CAD build for the part. Positions are in the model's coordinates, mm. Face numbers are marked on the shaded views. A direction names the side the tool comes from. Give positions to 0.01 mm unless a question says otherwise; leave off trailing zeros. Order: outer loops, then holes, each group sorted by start corner. A loop starts at its lowest first (then second) coordinate and runs counter-clockwise, first axis right, second up.
Item 1: Band-saw the part on A-A on x = -6. Give the cut face in (y, z), plus the area to 3 significant figures.
Item 2: Band-saw the part on D-D on x = 15.25. Give the cut face in (y, z).
Item 3: Which spindle directions (+Z, -Z, +X, -X, +Y, -Y) get a long thin tool onto all of the face, cutting with end or side? Do the marked faces 1, 2 and 3. Say none if no direction does.
Item 4: Flat gauge pins, fed straight in: P1, Ø3.5, axis at x = 15, z = 11.5, coming from the -Y side; P2, Ø2, axis at y = -12.5, z = 17.5, coming from the +X side; P3, Ø1.5, axis at x = 15.5, z = 18, coming from the +Y side. Where does each tip first touch, or does it go through?
Item 5: Wall check: L1, parallel to X at y = -0.25, z = 15.5; L2, parallel to X at y = -14.5, z = 23; L3, parallel to X at y = 0.25, z = 6.75. Give the ranges that are in metal, low to high.
Item 6: Band-saw the part on C-C on y = -11.5. Give the cut face in (x, z), plus the area to 3 significant figures.
Item 7: Band-saw the part on B-B on z = 8. Give the cut face in (x, y), plus the area to 3 significant figures.
```python
from build123d import *

# Parameters (mm, degrees)
F1_DEPTH = 25


with BuildPart() as f1:
    # F0 (on Top) → F1 (new body)
    with BuildSketch(Plane.XY):
        with BuildLine():
            ThreePointArc((0, -10.5), (-7.4246212025, 7.4246212025), (10.5, 0))
            Line((10.5, 0), (12, 0))
            ThreePointArc((12, 0), (-8.4852813742, 8.4852813742), (0, -12))
            Line((0, -12), (0, -10.5))
        make_face()
        with BuildLine():
            Line((12, 0), (10.5, 0))
            ThreePointArc((10.5, 0), (10.473041604, -0.7519305564), (10.3923048454, -1.5))
            Line((10.3923048454, -1.5), (11.9058808998, -1.5))
            ThreePointArc((11.9058808998, -1.5), (11.9764471108, -0.7514749505), (12, 0))
        make_face()
        with BuildLine():
            Line((17, 0), (12, 0))
            ThreePointArc((12, 0), (11.9764471108, -0.7514749505), (11.9058808998, -1.5))
            Line((11.9058808998, -1.5), (17, -1.5))
            Line((17, -1.5), (17, 0))
        make_face()
        with BuildLine():
            ThreePointArc((1.5, -10.3923048454), (0.7519305564, -10.473041604), (0, -10.5))
            Line((0, -10.5), (0, -12))
            ThreePointArc((0, -12), (0.7514749505, -11.9764471108), (1.5, -11.9058808998))
            Line((1.5, -11.9058808998), (1.5, -10.3923048454))
        make_face()
        with BuildLine():
            ThreePointArc((1.5, -11.9058808998), (0.7514749505, -11.9764471108), (0, -12))
            Line((0, -12), (0, -17))
            Line((0, -17), (1.5, -17))
            Line((1.5, -17), (1.5, -11.9058808998))
        make_face()
    extrude(amount=F1_DEPTH)


solid = f1.part
```
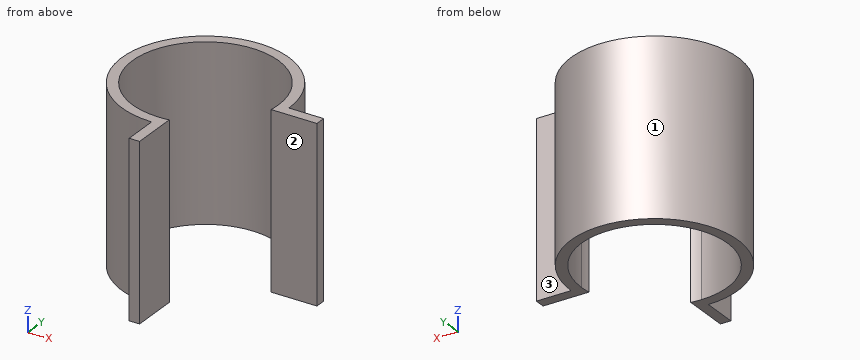
The answers:
1. outline: (-10.39, 0) - (-8.62, 0) - (-8.62, 25) - (-10.39, 25) - close; (8.62, 0) - (10.39, 0) - (10.39, 25) - (8.62, 25) - close
1. area: 88.8 mm2
2. outline: (-1.5, 0) - (0, 0) - (0, 25) - (-1.5, 25) - close
3. face 1: +Z, -Z
3. face 2: +Z, -Z, +X, -Y
3. face 3: +Z, -Z, +X, +Y
4. P1: stops at y = -1.5
4. P2: stops at x = 1.5
4. P3: stops at y = 0
5. L1: x = -12 to -10.5, 10.5 to 17
5. L2: x = 0 to 1.5
5. L3: x = -12 to -10.5, 10.5 to 12
6. outline: (-3.43, 0) - (1.5, 0) - (1.5, 25) - (-3.43, 25) - close
6. area: 123 mm2
7. outline: (0, -17) - (1.5, -17) - (1.5, -10.39) arc R10.5 cw (long way) to (10.39, -1.5) - (17, -1.5) - (17, 0) - (12, 0) arc R12 ccw (long way) to (0, -12) - close
7. area: 99.1 mm2
